Input: part model. Units: mm. Frame: model coordinates. Face numbers are marked on the shaded views. A direction names the side the tool comes from. Give positions to 0.01 mm unless a question says otherwise; leave off trailing zeros. Loops run counter-clockwise (first coordinate to the right, second up) from the corner with the lowest first, then second, coordinate; pieces in that order, holes last. Notation, with made-up numbers: M -2.5,-35 L 43.5,-35 A11 ccw 43.5,-23 Z; hole C 14.25,66 d3. An arc over 180 degrees is marked long. One line per item, written item: value. Start each with the question number.
(1) Pin query (flat end, axial travel): P1, Ø7.5, axis at x = -5, z = 38, coming from the +Y side. Return the tip coordinate at first contact, or that it passes through.
(2) Access query for the marked faces 1 and 2. Directions: +Z, -Z, +X, -X, +Y, -Y. A direction counts if a zero-diameter tool reaches every point of the face in a straight line with its end or side. Return the directions, or none.
(3) Section A-A on z = 4.5. Output: boundary loops of the cut face in (x, y).
(4) Section B-B on y = 31. Output: boundary loops of the cut face in (x, z), plus the area to 3 significant figures.
(5) Section C-C on x = 0.25. Output: boundary loops of the cut face in (y, z), plus the area to 3 significant figures.
(6) Pull-direction query (Y, two-part tool) for the marked faces 3, 4, 5 and 6; classes: released by +Y, released by -Y, zero draft, split by the parting line, or undercut.
(7) Ray query, line 1 along Y through (x, z) = (4, 4.5); line 2 along Z through (x, y) = (2, 31.5); line 3 along Z through (x, y) = (-2.25, 37.5). Return the intervals inside material, ascending. Write a range as from..to.
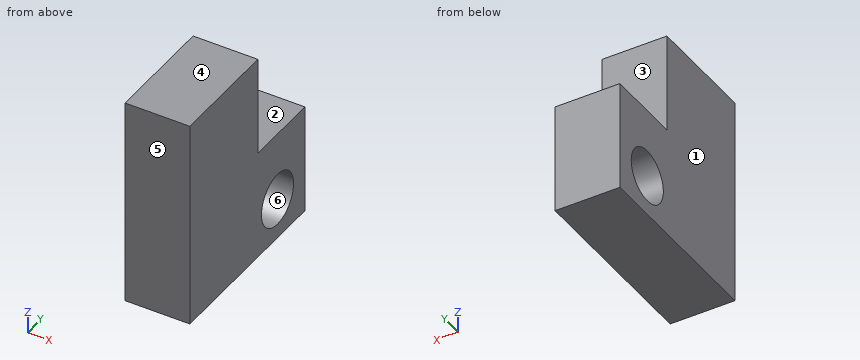
```python
from build123d import *

# Parameters (mm, degrees)
SKETCH1_W            = 42.5
SKETCH1_H            = 55.85
BOSS_EXTRUDE2_DEPTH  = 42.5
SKETCH5_R            = 3
CUT_EXTRUDE2_DEPTH   = 42.5
SKETCH6_W            = 42.5
SKETCH6_H            = 42.5
CUT_EXTRUDE3_DEPTH   = 39.5
SKETCH7_R            = 12
SKETCH7_R_2          = 1.5
CUT_EXTRUDE4_DEPTH   = 39.5
SKETCH9_W            = 10
SKETCH9_H            = 42.5
CUT_EXTRUDE5_DEPTH   = 39.5
CHAMFER1_SIZE        = 3
CHAMFER2_SIZE        = 2
SKETCH10_W           = 2
SKETCH10_H           = 2.21509362
BOSS_EXTRUDE3_DEPTH  = 3
SKETCH12_W           = 2
SKETCH12_H           = 3
BOSS_EXTRUDE4_DEPTH  = 3
BOSS_EXTRUDE5_DEPTH  = 2
BOSS_EXTRUDE6_DEPTH  = 2
SKETCH16_W           = 9
SKETCH16_H           = 9
SKETCH16_R           = 3.175
BOSS_EXTRUDE8_DEPTH  = 5
SKETCH17_R           = 3
CUT_EXTRUDE6_DEPTH   = 5
SKETCH18_W           = 9
SKETCH18_H           = 7.183282928
BOSS_EXTRUDE9_DEPTH  = 2
SKETCH19_R           = 3.175
CUT_EXTRUDE7_DEPTH   = 5
SKETCH20_W           = 36.5
SKETCH20_H           = 45.349147475
CUT_EXTRUDE9_DEPTH   = 66
CUT_EXTRUDE10_DEPTH  = 66
SKETCH22_R           = 12
SKETCH22_R_2         = 11.45
SKETCH22_R_3         = 1.5
SKETCH22_R_4         = 1.55
BOSS_EXTRUDE13_DEPTH = 3
SKETCH23_W           = 42.5
SKETCH23_H           = 7.46509362
CUT_EXTRUDE11_DEPTH  = 3
CHAMFER3_SIZE        = 2
SKETCH24_R           = 13.75
SKETCH24_R_2         = 11.45
BOSS_EXTRUDE14_DEPTH = 4
BOSS_EXTRUDE15_START = 10
SKETCH25_W           = 42.5
SKETCH25_H           = 33.508189308
SKETCH25_R           = 3.175
BOSS_EXTRUDE15_DEPTH = 10
CUT_EXTRUDE12_DEPTH  = 142
CHAMFER4_SIZE        = 10
SKETCH27_W           = 1.831902159
SKETCH27_H           = 1.026975453
BOSS_EXTRUDE16_DEPTH = 0.2
SKETCH28_R           = 3.175
BOSS_EXTRUDE17_DEPTH = 10
SKETCH29_R           = 6.15
BOSS_EXTRUDE19_DEPTH = 15
CUT_EXTRUDE13_DEPTH  = 50


with BuildPart() as part:
    # Sketch1 → Boss-Extrude2 (new body)
    with BuildSketch(Plane.XY):
        with Locations((-16.653499003, 3.960644895)):
            Rectangle(SKETCH1_W, SKETCH1_H)
    extrude(amount=BOSS_EXTRUDE2_DEPTH)

    # Sketch5 → Cut-Extrude2 (cut)
    with BuildSketch(Plane.XY.offset(42.5)):
        with Locations((-31.903499003, 25.965832134)):
            Circle(SKETCH5_R)
        with Locations(Location((-1.403499003, 25.965832134, 0), (0, 0, 180))):
            Circle(SKETCH5_R)
    extrude(amount=-CUT_EXTRUDE2_DEPTH, mode=Mode.SUBTRACT)

    # Sketch6 → Cut-Extrude3 (cut)
    with BuildSketch(Plane.ZY.offset(37.903499003)):
        with Locations((21.25, -0.499261485)):
            Rectangle(SKETCH6_W, SKETCH6_H)
    extrude(amount=-CUT_EXTRUDE3_DEPTH, mode=Mode.SUBTRACT)

    # Sketch7 → Cut-Extrude4 (cut)
    with BuildSketch(Plane(origin=(4.596500997, 0, 0), x_dir=(0, 0, -1), z_dir=(1, 0, 0))):
        with Locations((-21.25, -0.499261485)):
            Circle(SKETCH7_R)
        with Locations((-37, -16.249261485)):
            Circle(SKETCH7_R_2)
        with Locations((-5.5, -16.249261485)):
            Circle(SKETCH7_R_2)
        with Locations((-37, 14.750738515)):
            Circle(SKETCH7_R_2)
        with Locations((-5.5, 14.750738515)):
            Circle(SKETCH7_R_2)
    extrude(amount=-CUT_EXTRUDE4_DEPTH, mode=Mode.SUBTRACT)

    # Sketch9 → Cut-Extrude5 (cut)
    with BuildSketch(Plane.XZ.offset(23.964355105)):
        with Locations((-32.903499003, 21.25)):
            Rectangle(SKETCH9_W, SKETCH9_H)
    extrude(amount=-CUT_EXTRUDE5_DEPTH, mode=Mode.SUBTRACT)

    # Chamfer1
    chamfer1_edges = [part.edges().sort_by_distance(p)[0] for p in [
        (-37.903499003, 20.750738515, 21.25),
        (-37.903499003, 31.885644895, 21.25),
    ]]
    chamfer(chamfer1_edges, length=CHAMFER1_SIZE)

    # Chamfer2
    chamfer2_edges = [part.edges().sort_by_distance(p)[0] for p in [
        (4.596500997, -23.964355105, 21.25),
    ]]
    chamfer(chamfer2_edges, length=CHAMFER2_SIZE)

    # Sketch10 → Boss-Extrude3 (add)
    with BuildSketch(Plane.ZY.offset(27.903499003)):
        with Locations((43.5, -22.856808295)):
            Rectangle(SKETCH10_W, SKETCH10_H)
        with Locations((-1, -22.856808295)):
            Rectangle(SKETCH10_W, SKETCH10_H)
    extrude(amount=-BOSS_EXTRUDE3_DEPTH)

    # Sketch12 → Boss-Extrude4 (add)
    with BuildSketch(Plane.ZY.offset(-1.596500997)):
        with Locations((43.5, 19.250738515)):
            Rectangle(SKETCH12_W, SKETCH12_H)
        with Locations((-1, 19.250738515)):
            Rectangle(SKETCH12_W, SKETCH12_H)
    extrude(amount=-BOSS_EXTRUDE4_DEPTH)

    # Sketch13 → Boss-Extrude5 (add)
    with BuildSketch(Plane(origin=(0, 0, -2), x_dir=(-1, 0, 0), z_dir=(0, 0, -1))):
        Polygon((-1.596500997, 17.750738515), (24.903499003, -21.749261485), (27.903499003, -21.749261485), (-1.596500997, 20.750738515), align=None)
    extrude(amount=-BOSS_EXTRUDE5_DEPTH)

    # Sketch14 → Boss-Extrude6 (add)
    with BuildSketch(Plane.XY.offset(44.5)):
        Polygon((1.596500997, 17.750738515), (-24.903499003, -21.749261485), (-27.903499003, -21.749261485), (1.596500997, 20.750738515), align=None)
    extrude(amount=-BOSS_EXTRUDE6_DEPTH)

    # Sketch16 → Boss-Extrude8 (add)
    # profile 1 of 2: a face of its own
    with BuildSketch(Plane(origin=(4.596500997, 0, 0), x_dir=(0, 0, -1), z_dir=(1, 0, 0))):
        with Locations((-38, 34.568927823)):
            Rectangle(SKETCH16_W, SKETCH16_H)
        with Locations((-38, 34.568927823)):
            Circle(SKETCH16_R, mode=Mode.SUBTRACT)
    # profile 2 of 2: a face of its own
    with BuildSketch(Plane(origin=(4.596500997, 0, 0), x_dir=(0, 0, -1), z_dir=(1, 0, 0))):
        with Locations((-4.5, 34.568927823)):
            Rectangle(SKETCH16_W, SKETCH16_H)
        with Locations((-4.5, 34.568927823)):
            Circle(SKETCH16_R, mode=Mode.SUBTRACT)
    extrude(amount=-BOSS_EXTRUDE8_DEPTH)

    # Sketch17 → Cut-Extrude6 (cut)
    with BuildSketch(Plane(origin=(4.596500997, 0, 0), x_dir=(0, 0, -1), z_dir=(1, 0, 0))):
        with Locations((-38, 34.568927823)):
            Circle(SKETCH17_R)
        with Locations((-4.5, 34.568927823)):
            Circle(SKETCH17_R)
    extrude(amount=-CUT_EXTRUDE6_DEPTH, mode=Mode.SUBTRACT)

    # Sketch18 → Boss-Extrude9 (add)
    with BuildSketch(Plane.ZY.offset(0.403499003)):
        with Locations((4.5, 35.477286359)):
            Rectangle(SKETCH18_W, SKETCH18_H)
        with Locations((38, 35.477286359)):
            Rectangle(SKETCH18_W, SKETCH18_H)
    extrude(amount=BOSS_EXTRUDE9_DEPTH)

    # Sketch19 → Cut-Extrude7 (cut)
    with BuildSketch(Plane(origin=(4.596500997, 0, 0), x_dir=(0, 0, -1), z_dir=(1, 0, 0))):
        with Locations((-38, 34.568927823)):
            Circle(SKETCH19_R)
        with Locations(Location((-4.5, 34.568927823, 0), (0, 0, 180))):
            Circle(SKETCH19_R)
    extrude(amount=-CUT_EXTRUDE7_DEPTH, mode=Mode.SUBTRACT)

    # Sketch20 → Cut-Extrude9 (cut, symmetric)
    with BuildSketch(Plane.XY.offset(42.5)):
        with Locations((-16.653499003, -1.923835222)):
            Rectangle(SKETCH20_W, SKETCH20_H)
    extrude(amount=CUT_EXTRUDE9_DEPTH, both=True, mode=Mode.SUBTRACT)

    # Sketch21 → Cut-Extrude10 (cut, symmetric)
    with BuildSketch(Plane(origin=(4.596500997, 0, 0), x_dir=(0, 0, -1), z_dir=(1, 0, 0))):
        Polygon((0, 39.068927823), (0, -21.964355105), (2.461652374, -21.964355105), (3.037977258, 39.068927823), (0.568013469, 39.068927823), align=None)
        Polygon((-42.5, 39.068927823), (-42.5, -21.964355105), (-44.961652374, -21.964355105), (-45.537977258, 39.068927823), (-43.068013469, 39.068927823), align=None)
    extrude(amount=CUT_EXTRUDE10_DEPTH, both=True, mode=Mode.SUBTRACT)

    # Sketch22 → Boss-Extrude13 (add)
    # profile 1 of 5: a face of its own
    with BuildSketch(Plane(origin=(4.596500997, 0, 0), x_dir=(0, 0, -1), z_dir=(1, 0, 0))):
        with Locations((-21.25, -0.499261485)):
            Circle(SKETCH22_R)
        with Locations((-21.25, -0.499261485)):
            Circle(SKETCH22_R_2, mode=Mode.SUBTRACT)
    # profile 2 of 5: a face of its own
    with BuildSketch(Plane(origin=(4.596500997, 0, 0), x_dir=(0, 0, -1), z_dir=(1, 0, 0))):
        with Locations((-37, 14.750738515)):
            Circle(SKETCH22_R_3)
    # profile 3 of 5: a face of its own
    with BuildSketch(Plane(origin=(4.596500997, 0, 0), x_dir=(0, 0, -1), z_dir=(1, 0, 0))):
        with Locations((-5.524563877, 14.750738515)):
            Circle(SKETCH22_R_4)
    # profile 4 of 5: a face of its own
    with BuildSketch(Plane(origin=(4.596500997, 0, 0), x_dir=(0, 0, -1), z_dir=(1, 0, 0))):
        with Locations((-5.5, -16.249261485)):
            Circle(SKETCH22_R_3)
    # profile 5 of 5: a face of its own
    with BuildSketch(Plane(origin=(4.596500997, 0, 0), x_dir=(0, 0, -1), z_dir=(1, 0, 0))):
        with Locations((-37, -16.249261485)):
            Circle(SKETCH22_R_3)
    extrude(amount=-BOSS_EXTRUDE13_DEPTH)

    # Sketch23 → Cut-Extrude11 (cut)
    with BuildSketch(Plane(origin=(4.596500997, 0, 0), x_dir=(0, 0, -1), z_dir=(1, 0, 0))):
        with Locations((-21.25, -20.231808295)):
            Rectangle(SKETCH23_W, SKETCH23_H)
    extrude(amount=-CUT_EXTRUDE11_DEPTH, mode=Mode.SUBTRACT)

    # Chamfer3
    chamfer3_edges = [part.edges().sort_by_distance(p)[0] for p in [
        (4.596500997, -16.499261485, 21.25),
    ]]
    chamfer(chamfer3_edges, length=CHAMFER3_SIZE)

    # Sketch24 → Boss-Extrude14 (add)
    with BuildSketch(Plane.ZY.offset(-1.596500997)):
        with Locations(Location((21.25, -0.499261485, 0), (0, 0, 180))):
            Circle(SKETCH24_R)
        with Locations(Location((21.25, -0.499261485, 0), (0, 0, 180))):
            Circle(SKETCH24_R_2, mode=Mode.SUBTRACT)
    extrude(amount=BOSS_EXTRUDE14_DEPTH)

    # Sketch25 → Boss-Extrude15 (add)
    with BuildSketch(Plane(origin=(4.596500997, 0, 0), x_dir=(0, 0, -1), z_dir=(1, 0, 0)).offset(BOSS_EXTRUDE15_START)):
        with Locations((-21.25, 22.314833169)):
            Rectangle(SKETCH25_W, SKETCH25_H)
        with Locations((-38, 34.568927823)):
            Circle(SKETCH25_R, mode=Mode.SUBTRACT)
        with Locations((-4.5, 34.568927823)):
            Circle(SKETCH25_R, mode=Mode.SUBTRACT)
    extrude(amount=-BOSS_EXTRUDE15_DEPTH)

    # Sketch26 → Cut-Extrude12 (cut)
    with BuildSketch(Plane(origin=(0, 0, 0), x_dir=(-1, 0, 0), z_dir=(0, 0, -1))):
        Polygon((-4.596500997, 39.068927823), (-4.596500997, -17.856619688), (37.419914356, -17.856619688), (42.573197426, 39.068927823), align=None)
    extrude(amount=-CUT_EXTRUDE12_DEPTH, mode=Mode.SUBTRACT)

    # Chamfer4
    chamfer4_edges = [part.edges().sort_by_distance(p)[0] for p in [
        (9.596500997, 5.560738515, 42.5),
        (9.596500997, 5.560738515, 0),
    ]]
    chamfer(chamfer4_edges, length=CHAMFER4_SIZE)

    # Sketch27 → Boss-Extrude16 (add)
    with BuildSketch(Plane.XZ.offset(-5.560738515)):
        with Locations((11.95576893, 21.763487727)):
            Rectangle(SKETCH27_W, SKETCH27_H)
    extrude(amount=BOSS_EXTRUDE16_DEPTH)

    # Sketch28 → Boss-Extrude17 (add)
    with BuildSketch(Plane(origin=(14.596500997, 0, 0), x_dir=(0, 0, -1), z_dir=(1, 0, 0))):
        Polygon((-42.578884897, 40.068927823), (0, 40.068927823), (1, 40.068927823), (1, 15.146524953), (-8.635786438, 5.510738515), (-33.864213562, 5.510738515), (-43.5, 15.146524953), (-43.5, 40.068927823), align=None)
        with Locations((-38, 34.568927823)):
            Circle(SKETCH28_R, mode=Mode.SUBTRACT)
        with Locations((-4.5, 34.568927823)):
            Circle(SKETCH28_R, mode=Mode.SUBTRACT)
    extrude(amount=-BOSS_EXTRUDE17_DEPTH)

    # Sketch29 → Boss-Extrude19 (add)
    with BuildSketch(Plane.ZY.offset(-4.596500997)):
        Polygon((-5, 45.068927823), (-5, 1.010738515), (43.772310913, 1.010738515), (43.772310913, 27.051079093), (20.597179394, 27.051079093), (20.597179394, 45.068927823), align=None)
        with Locations(Location((4.5, 34.568927823, 0), (0, 0, 153.419803228))):
            Circle(SKETCH29_R, mode=Mode.SUBTRACT)
    extrude(amount=BOSS_EXTRUDE19_DEPTH)

    # Sketch30 → Cut-Extrude13 (cut)
    with BuildSketch(Plane.XY.offset(43.772310913)):
        Polygon((4.596500997, 40.068927823), (4.596500997, 5.510738515), (14.596500997, 4.365687142), (14.596500997, 40.068927823), align=None)
    extrude(amount=-CUT_EXTRUDE13_DEPTH, mode=Mode.SUBTRACT)


solid = part.part
```
Output values:
1. P1: stops at y = 27.05
2. face 1: +Z, -Z, -X, +Y, -Y
2. face 2: +Z, +X, -X, +Y
3. outline: M -10.4,1.01 L 4.6,1.01 L 4.6,28.42 L -10.4,28.42 Z; M -10.4,40.72 L 4.6,40.72 L 4.6,45.07 L -10.4,45.07 Z
4. outline: M -10.4,-5 L 4.6,-5 L 4.6,-0.51 L -10.4,-0.51 Z; M -10.4,9.51 L 4.6,9.51 L 4.6,20.6 L -10.4,20.6 Z
4. area: 234 mm²
5. outline: M 1.01,-5 L 45.07,-5 L 45.07,20.6 L 27.05,20.6 L 27.05,43.77 L 1.01,43.77 Z; hole C 34.57,4.5 d12.3
5. area: 1,610 mm²
6. face 3: released by +Y
6. face 4: zero draft
6. face 5: released by -Y
6. face 6: undercut
7. line 1: y = 1.01..28.42, 40.72..45.07
7. line 2: z = -5..-0.83, 9.83..20.6
7. line 3: z = -5..-0.91, 9.91..20.6
